Input: dimensioned drawing with shaded views. Units: mm. Origin: part minimum x, y, z. A direction names the side the tool comes from. Round coordinates to 2 decimals unless told otherwise and drop trailing zeros. Order: outer loops, then holes, each group sorted by start corner. A loop starts at its lowest first (then second) coordinate and runs counter-clockwise, first axis right, second up. Notation, with made-up numbers: (83.5, -34.75) - (89.5, -34.75) arc R19 ccw to (89.5, -22.75) - close; hole circle Ø5 at (26.5, 50.25). An arc over 180 degrees is marked (long way). Return JSON: item names as keys, results as strings. Group by question number.
1) Ray query, line 1 (Y direction, x = 44, z = 39); line 2 (Z direction, x = 41, y = 23); line 3 (Z direction, x = 43, y = 70.5) (1 decimal). Return the intervals inside material, ascending. Write a range as from..to.
2) Section C-C, the plane y = 36. Return loops of the section in (x, z), plus the area to 3 significant figures.
3) Contact query for a flat-ended pin moving along its axis: P1, Ø5, axis at y = 74, z = 140.5, coming from the -X side. Output: stop coordinate, or through.
4) Access query for the marked faces 1 and 2. Directions: +Z, -Z, +X, -X, +Y, -Y. A direction counts if a zero-diameter tool reaches every point of the face in a straight line with its end or side. Return the directions, or none.
5) Section B-B, the plane x = 15. Give the number of separate pieces and of enclosed holes in the cut face.
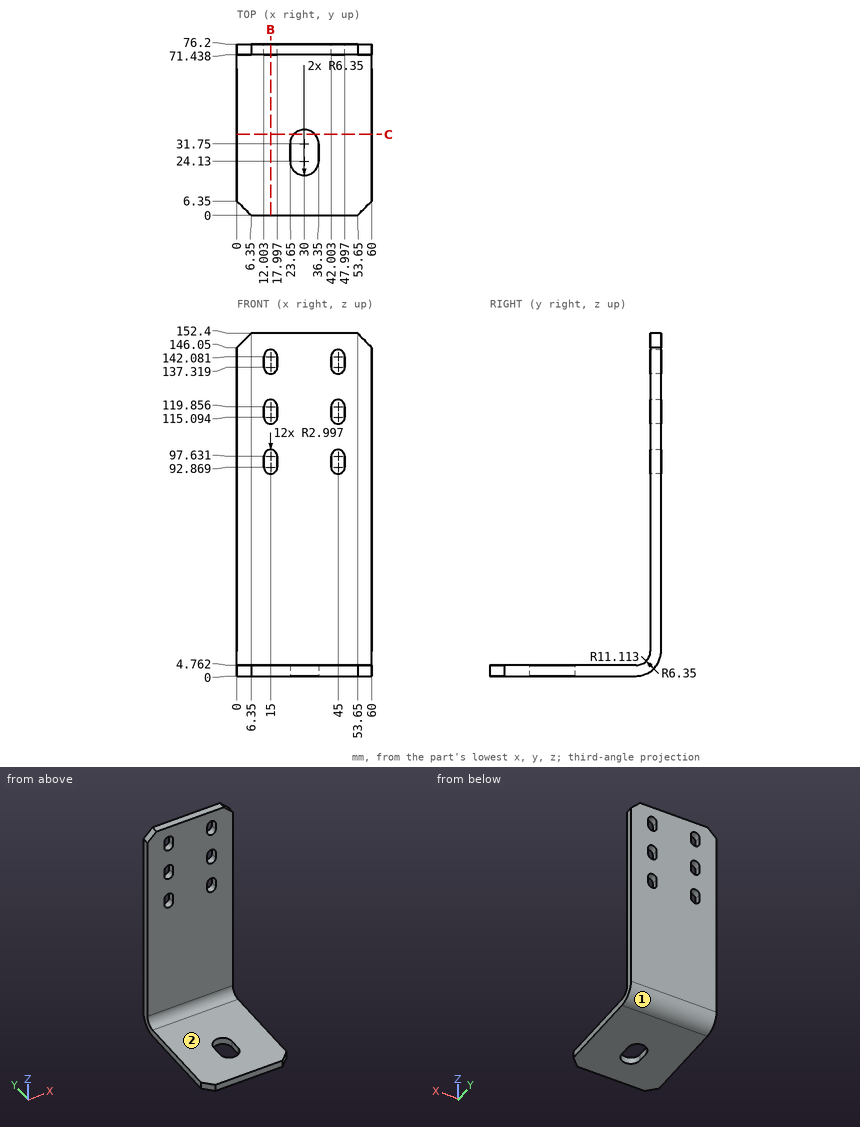
Geometry check:
{
 "1": {"line 1": "71.44..76.2", "line 2": "0..4.76", "line 3": "1.4..7.8"},
 "2": {"outline": "(0, 0) - (25.28, 0) - (25.28, 4.76) - (0, 4.76) - close; (34.72, 0) - (60, 0) - (60, 4.76) - (34.72, 4.76) - close", "area": "241 mm2"},
 "3": {"P1": "x = 0"},
 "4": {"face 1": "-Z, +X, -X, +Y", "face 2": "+Z, +X, -X, -Y"},
 "5": {"separate pieces": "4", "enclosed holes": "0"}
}
